Geometry check sheet. Reference: the model listing, model coordinates, mm. Coordinates: 2 decimals unless noted, no trailing zeros. Loops run counter-clockwise (first coordinate to the right, second up) from the corner with the lowest first, then second, coordinate; pieces in that order, holes last. Notation, with made-up numbers: (-15, 59) - (31, 59) arc R10 cw to (31, 68) - close; hole circle Ø5 at (81.25, -6). An arc over 180 degrees is marked (long way). Write each question's results on one line, items separated by ' | '. Start each with the question number.
(1) Material ranges on probe 1 along Z at (x, y) = (-1.5, 1.3); probe 2 along Z at (x, y) = (1, 1.25); probe 3 along X at (y, z) = (-0.2, -3), recorded low to high.
(2) Go/stop test with flat-tipped pins: pin 1 Ø3 at (x, y) = (-2.5, 2.5) entering from +Z; pin 2 Ø1 at (x, z) = (2.5, -7.5) entering from -Y; pin 3 Ø3 at (x, y) = (2, -2) entering from -Z. Record where each tip stops, or that it passes through.
(3) Sectioned sample at B-B (x = 0). Enter the section's corners in (y, z), plus the area to 3 significant figures.
(4) Sectioned sample at A-A (z = 42.5). Enter the section's corners in (x, y).
(5) Sectioned sample at C-C (z = -15). Enter the section's corners in (x, y).
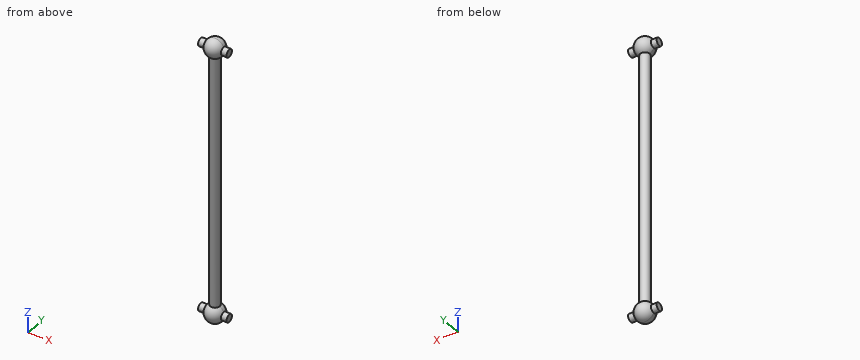
from build123d import *
from build123d.topology import SkipClean

# Parameters (mm, degrees)
BOSS_EXTRUDE1_DEPTH      = 42.5
BOSS_EXTRUDE1_DEPTH_BACK = 42.5
SKETCH1_R                = 1.5
SKETCH3_R                = 1.25
BOSS_EXTRUDE2_DEPTH      = 4.5


with BuildPart() as part:
    # Sketch1 → Boss-Extrude1 (new, two sides: drawn at the far end of the back side and taken through both)
    with BuildSketch(Plane.XY.offset(-BOSS_EXTRUDE1_DEPTH_BACK)):
        Circle(SKETCH1_R)
    extrude(amount=BOSS_EXTRUDE1_DEPTH + BOSS_EXTRUDE1_DEPTH_BACK)

    # Sketch2 → Revolve1 (revolve)
    with SkipClean():  # the faces are left unmerged after this step: merging them gives an invalid solid
        with BuildSketch(Plane(origin=(0, 0, 0), x_dir=(0, 0, -1), z_dir=(1, 0, 0))):
            with BuildLine():
                ThreePointArc((-39.5, 0), (-40.378679656, 2.121320344), (-42.5, 3))
                Line((-42.5, 3), (-42.5, -3))
                ThreePointArc((-42.5, -3), (-40.378679656, -2.121320344), (-39.5, 0))
            make_face()
            with BuildLine():
                Line((-42.5, -3), (-42.5, 3))
                ThreePointArc((-42.5, 3), (-45.5, 0), (-42.5, -3))
            make_face()
        revolve1 = revolve(axis=Axis((0, 3, 42.5), (0, -1, 0)))

    # Sketch3 → Boss-Extrude2 (add, symmetric)
    with SkipClean():  # the faces are left unmerged after this step: merging them gives an invalid solid
        with BuildSketch(Plane(origin=(0, 0, 0), x_dir=(0, 0, -1), z_dir=(1, 0, 0))):
            with Locations((-42.5, 0)):
                Circle(SKETCH3_R)
        boss_extrude2 = extrude(amount=BOSS_EXTRUDE2_DEPTH, both=True)

    # Mirror1: Revolve1, Boss-Extrude2 across plane
    with SkipClean():  # the faces are left unmerged after this step: merging them gives an invalid solid
        add(revolve1.mirror(Plane.XY))
        add(boss_extrude2.mirror(Plane.XY))


solid = part.part
Outcome:
1) probe 1: z = -44.75 to -40.25, 40.25 to 44.75 | probe 2: z = -45.04 to -39.96, 39.96 to 45.04 | probe 3: x = -1.49 to 1.49
2) pin 1: stops at z = 44.7 | pin 2: passes through | pin 3: stops at z = -45.19
3) outline: (-1.5, -39.9) arc R3 ccw (long way) to (1.5, -39.9) - (1.5, 39.9) arc R3 ccw (long way) to (-1.5, 39.9) - close | area: 294 mm2
4) outline: (-4.5, -1.25) - (-2.73, -1.25) arc R3 ccw to (2.73, -1.25) - (4.5, -1.25) - (4.5, 1.25) - (2.73, 1.25) arc R3 ccw to (-2.73, 1.25) - (-4.5, 1.25) - close
5) outline: circle Ø3 at (0, 0)
